Check sheet for the drawn part. Datum: minimum x, y, z corner. Units: mm. A direction names the side the tool comes from. Give positions to 0.01 mm unless a question says otherwise; leave off trailing zeros. Loops run counter-clockwise (first coordinate to the right, second up) from the corner with the lowest first, then second, coordinate; pieces in that order, holes last. Notation, with made-up numbers: M 74,38 L 87,38 A13 cw 87,46 Z; hole C -37,9.5 d4. An arc over 180 degrees is marked long. Write each question's results on one line, items separated by ' | '. Start each with the question number.
1. Sectioned sample at D-D on x = 25. Record the cut outline in (y, z).
2. Go/stop test with flat-tipped pins: pin 1 (8 mm diameter, centred on y = 17.5, z = 14, fed in from +X); pin 2 (12 mm diameter, centred on y = 12, z = 3.5, fed in from -X); pin 3 (6 mm diameter, centred on x = 24.5, z = 6, fed in from +Y). Record where each tip stops, or that it passes through.
3. Sectioned sample at A-A on y = 11. Record the cut outline in (x, z).
4. Material ranges on line 1 along X through (y, z) = (9.5, 3.25); line 2 along Y through (x, z) = (12.5, 9.25); line 3 along Z through (x, y) = (5.5, 19.5), recorded low to high.
5. Sectioned sample at C-C on y = 19.25. Record the cut outline in (x, z).
6. Sectioned sample at B-B on z = 6. Record the cut outline in (x, y), and give its area (3 significant figures).
7. Tool access check on the marked faces 1 and 2. Record the directions out of +Z, -Z, +X, -X, +Y, -Y that give a thin tool (end or side, any length) a straight path to the whole face; none if there is none.
8. Draft check along X on the marked faces 3, 4 and 5. Enter one of: pulls with the +X half, pulls with the -X half, needs draft (parallel to the pull), parting line crosses it, or undercut.
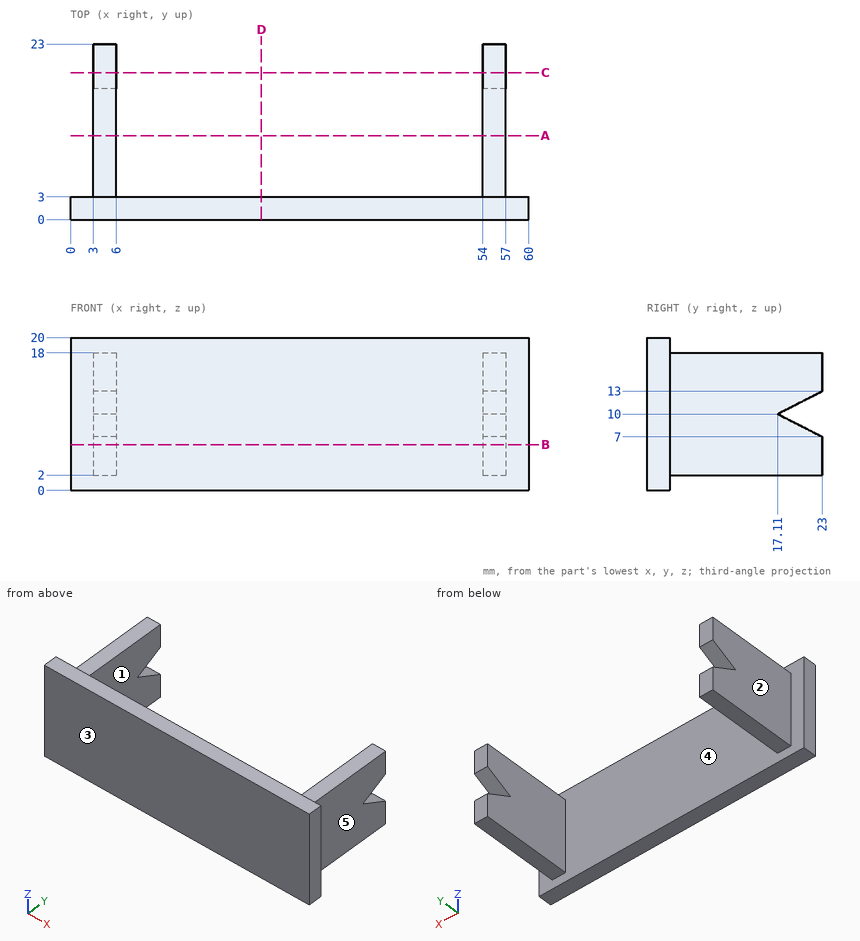
Output values:
1) outline: M 0,0 L 3,0 L 3,20 L 0,20 Z
2) pin 1: x = 57 | pin 2: x = 3 | pin 3: y = 3
3) outline: M 3,2 L 6,2 L 6,18 L 3,18 Z; M 54,2 L 57,2 L 57,18 L 54,18 Z
4) line 1: 3 to 6, 54 to 57 | line 2: 0 to 3 | line 3: 2 to 8.78, 11.22 to 18
5) outline: M 3,2 L 6,2 L 6,8.91 L 3,8.91 Z; M 3,11.09 L 6,11.09 L 6,18 L 3,18 Z; M 54,2 L 57,2 L 57,8.91 L 54,8.91 Z; M 54,11.09 L 57,11.09 L 57,18 L 54,18 Z
6) outline: M 0,0 L 60,0 L 60,3 L 57,3 L 57,23 L 54,23 L 54,3 L 6,3 L 6,23 L 3,23 L 3,3 L 0,3 Z | area: 300 mm2
7) face 1: +Z, -Z, +Y | face 2: +Z, -Z, -X, +Y
8) face 3: needs draft | face 4: undercut | face 5: pulls with the +X half
